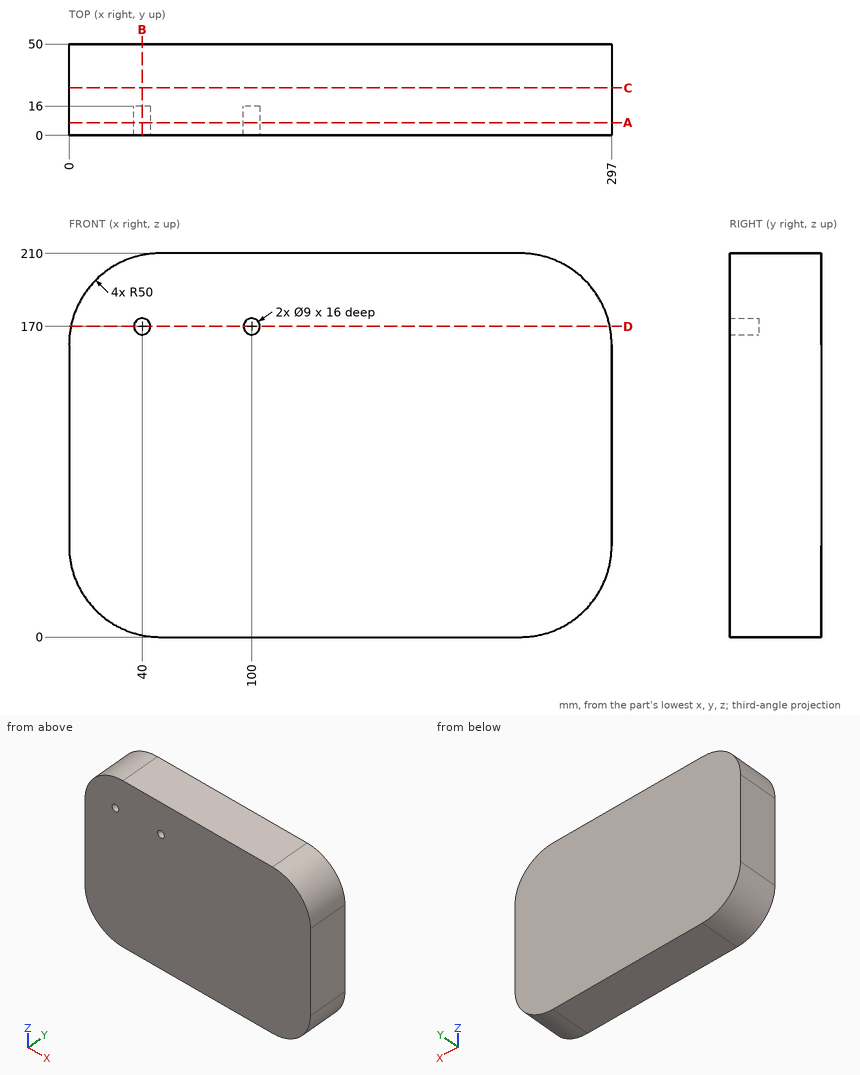
Job drawing, mm, ordinate dimensions from the low corner. One solid piece. Give positions to 0.01 mm unless a question says otherwise; leave off trailing zeros. Loops run counter-clockwise (first coordinate to the right, second up) from the corner with the lowest first, then second, coordinate; pieces in that order, holes last. Notation, with made-up numbers: M 31,17 L 79,17 A15 ccw 79,35 Z; hole C -4,12 d10. An arc over 180 degrees is marked long. Answer in a Markdown table with one row per item. Add a question column.
Item 1: Band-saw the part on A-A on y = 7. Give the cut face in (x, z), then the cut area to 3 significant figures.
Item 2: Band-saw the part on D-D on z = 170. Give the cut face in (x, y).
Item 3: Band-saw the part on C-C on y = 26. Give the cut face in (x, z), then the cut area to 3 significant figures.
Item 4: Drop a flat-ended pin along its axis: P1, Ø4.5, axis at x = 38.5, z = 169.5, coming from the -Y side. Give the stop position or say it passes through.
Item 5: Band-saw the part on B-B on x = 40. Give the cut face in (y, z).
Item 6: Probe probe 1 along Z at (x, y) = (100, 9.75); probe 2 along X at (y, z) = (9, 170); probe 3 along X at (y, z) = (48, 14). List the from-to ranges inside material, lowest first.
Reply:
| question | item | result |
|---|---|---|
| 1 | outline | M 0,50 A50 ccw 50,0 L 247,0 A50 ccw 297,50 L 297,160 A50 ccw 247,210 L 50,210 A50 ccw 0,160 Z; hole C 40,170 d9; hole C 100,170 d9 |
| 1 | area | 60,100 mm^2 |
| 2 | outline | M 1.01,0 L 35.5,0 L 35.5,16 L 44.5,16 L 44.5,0 L 95.5,0 L 95.5,16 L 104.5,16 L 104.5,0 L 295.99,0 L 295.99,50 L 1.01,50 Z |
| 3 | outline | M 0,50 A50 ccw 50,0 L 247,0 A50 ccw 297,50 L 297,160 A50 ccw 247,210 L 50,210 A50 ccw 0,160 Z |
| 3 | area | 60,200 mm^2 |
| 4 | P1 | stops at y = 16 |
| 5 | outline | M 0,1.01 L 50,1.01 L 50,208.99 L 0,208.99 L 0,174.5 L 16,174.5 L 16,165.5 L 0,165.5 Z |
| 6 | probe 1 | z = 0 to 165.5, 174.5 to 210 |
| 6 | probe 2 | x = 1.01 to 35.5, 44.5 to 95.5, 104.5 to 295.99 |
| 6 | probe 3 | x = 15.3 to 281.7 |
